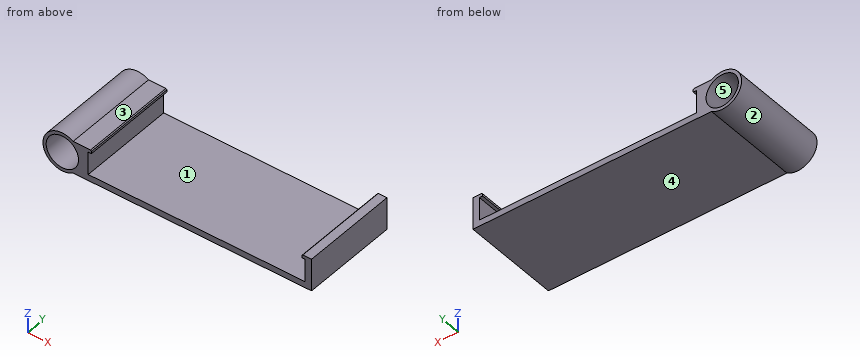
```python
from build123d import *

# Parameters (mm, degrees)
F0_R     = 5
F1_DEPTH = 30
F2_SIZE  = 0.3


with BuildPart() as f1:
    # F0 (on Front) → F1 (new body)
    with BuildSketch(Plane.XZ):
        with BuildLine():
            Line((3, 0), (0, 0))
            Line((0, 0), (-2.683375, 0))
            ThreePointArc((-2.683375, 0), (-12, -5), (-2.683375, -10))
            Line((-2.683375, -10), (0, -10))
            Line((0, -10), (71.1, -10))
            Line((71.1, -10), (71.1, 0))
            Line((71.1, 0), (68.1, 0))
            Line((68.1, 0), (68.1, -1))
            Line((68.1, -1), (69.1, -1))
            Line((69.1, -1), (69.1, -8.1))
            Line((69.1, -8.1), (2, -8.1))
            Line((2, -8.1), (2, -1))
            Line((2, -1), (3, -1))
            Line((3, -1), (3, 0))
        make_face()
        with Locations((-6, -5)):
            Circle(F0_R, mode=Mode.SUBTRACT)
    extrude(amount=F1_DEPTH)

    # F2
    f2_edges = [f1.edges().sort_by_distance(p)[0] for p in [
        (68.1, -15, 0),
        (3, -15, 0),
    ]]
    chamfer(f2_edges, length=F2_SIZE)


solid = f1.part
```
The model under review builds one solid part; all positions refer to its coordinate system, in mm. Face numbers are marked on the shaded views. A direction names the side the tool comes from. Round coordinates to 2 decimals unless told otherwise and drop trailing zeros. Order: outer loops, then holes, each group sorted by start corner. A loop starts at its lowest first (then second) coordinate and runs counter-clockwise, first axis right, second up. Notation, with made-up numbers: M -2,37 L 49,37 A22 cw 49,71 Z; hole C 80,23.25 d3. An arc over 180 degrees is marked long. Use a Markdown table: item, result.
1) Insertion check: pin 1 (0.8 mm diameter, centred on x = 68.5, y = -13, fed in from -Z); pin 2 (1.5 mm diameter, centred on x = 20.5, y = -13, fed in from +Z); pin 3 (2 mm diameter, centred on x = 70, y = -8.5, fed in from +Z). Each pin has a flat end and moves straight along its axis. Give the tip position at first contact, or say it passes through.
Report:
| item | result |
|---|---|
| pin 1 | z = -10 |
| pin 2 | z = -8.1 |
| pin 3 | z = 0 |
2) Consider section D-D (x = 49.5). Write out the cut boundary in (y, z).
Report:
| item | result |
|---|---|
| outline | M -30,-10 L 0,-10 L 0,-8.1 L -30,-8.1 Z |
3) Wall thickness on line 1 along X through (y, z) = (-20.25, -5.25); line 2 along Z through (x, y) = (-6, -21); line 3 along X through (y, z) = (-26, -0.5): over which ranges is each line inside the solid? List them lowest first. Write a range as [from, to].
Report:
| item | result |
|---|---|
| line 1 | [-11.99, -10.99], [-1.01, 2], [69.1, 71.1] |
| line 2 | [-11, -10], [0, 1] |
| line 3 | [-9.97, -8.18], [-3.82, 3], [68.1, 71.1] |
4) Consider section C-C (y = -7.25). Write out the cut boundary in (x, z).
Report:
| item | result |
|---|---|
| outline | M -2.68,-10 L 71.1,-10 L 71.1,0 L 68.4,0 L 68.1,-0.3 L 68.1,-1 L 69.1,-1 L 69.1,-8.1 L 2,-8.1 L 2,-1 L 3,-1 L 3,-0.3 L 2.7,0 L -2.68,0 A6 ccw long Z; hole C -6,-5 d10 |
5) Tool access review of the marked faces 4 and 5: name each direction out of +Z, -Z, +X, -X, +Y, -Y from which nothing blocks a thin tool from reaching the whole face with its end or side.
Report:
| item | result |
|---|---|
| face 4 | -Z, +X, +Y, -Y |
| face 5 | +Y, -Y |
6) Consider section B-B (z = -5). Write out the cut boundary in (x, y).
Report:
| item | result |
|---|---|
| outline | M -12,-30 L -11,-30 L -11,0 L -12,0 Z; M -1,-30 L 2,-30 L 2,0 L -1,0 Z; M 69.1,-30 L 71.1,-30 L 71.1,0 L 69.1,0 Z |
7) Draft analysis for pull direction X (two halves, no side actions). For the marked faces 1, 2 and 3, state which applies: released by +X, released by -X, zero draft, split by the parting line, or undercut.
Report:
| item | result |
|---|---|
| face 1 | undercut |
| face 2 | split by the parting line |
| face 3 | zero draft |
8) Consider section A-A (x = -6). Write out the cut boundary in (y, z), then the cut area to 3 significant figures.
Report:
| item | result |
|---|---|
| outline | M -30,-11 L 0,-11 L 0,-10 L -30,-10 Z; M -30,0 L 0,0 L 0,1 L -30,1 Z |
| area | 60.0 mm^2 |
